Check sheet for the modelled part. Datum: model origin and axes. Units: mm. Face numbers are marked on the shaded views. A direction names the side the tool comes from. Give positions to 0.01 mm unless a question says otherwise; leave off trailing zeros. Order: outer loops, then holes, each group sorted by start corner. A loop starts at its lowest first (then second) coordinate and runs counter-clockwise, first axis right, second up. Notation, with made-up numbers: (9, -7) -> (46, -7) arc R15 cw to (46, -3) -> close; hole circle Ø4 at (15, 14.5). An arc over 180 degrees is marked (long way). One line per question, with ' | ' between items. Start each with the question number.
from build123d import *

# Parameters (mm, degrees)
BOSS_EXTRUDE1_DEPTH = 3
CUT_EXTRUDE1_REACH  = 5
SKETCH3_W           = 2.8
SKETCH3_H           = 2.8


with BuildPart() as part:
    # Sketch1 → Boss-Extrude1 (new body)
    with BuildSketch(Plane(origin=(0, 0, 0), x_dir=(1, 0, 0), z_dir=(0, 1, 0))):
        Polygon((0, 14.43375673), (-12.5, -7.216878365), (12.5, -7.216878365), align=None)
    extrude(amount=BOSS_EXTRUDE1_DEPTH)

    # Sketch3 → Cut-Extrude1 (cut, up to next)
    with BuildSketch(Plane(origin=(0, 3, 0), x_dir=(1, 0, 0), z_dir=(0, 1, 0)), mode=Mode.PRIVATE) as cut_extrude1_sk1:
        Polygon((6.95, 2.396003617), (4.525128869, 0.996003617), (3.125128869, 3.420874748), (5.55, 4.820874748), align=None)
    cut_extrude1_tool1 = extrude(cut_extrude1_sk1.sketch, amount=-CUT_EXTRUDE1_REACH, mode=Mode.PRIVATE) & part.part
    add(cut_extrude1_tool1.solids().sort_by_distance((5.037564, 3, -2.908439))[0], mode=Mode.SUBTRACT)
    # Sketch3 → Cut-Extrude1 (cut, up to next)
    with BuildSketch(Plane(origin=(0, 3, 0), x_dir=(1, 0, 0), z_dir=(0, 1, 0)), mode=Mode.PRIVATE) as cut_extrude1_sk2:
        Polygon((-6.95, 2.396003617), (-4.525128869, 0.996003617), (-3.125128869, 3.420874748), (-5.55, 4.820874748), align=None)
    cut_extrude1_tool2 = extrude(cut_extrude1_sk2.sketch, amount=-CUT_EXTRUDE1_REACH, mode=Mode.PRIVATE) & part.part
    add(cut_extrude1_tool2.solids().sort_by_distance((-5.037564, 3, -2.908439))[0], mode=Mode.SUBTRACT)
    # Sketch3 → Cut-Extrude1 (cut, up to next)
    with BuildSketch(Plane(origin=(0, 3, 0), x_dir=(1, 0, 0), z_dir=(0, 1, 0)), mode=Mode.PRIVATE) as cut_extrude1_sk3:
        with Locations((0, -5.816878365)):
            Rectangle(SKETCH3_W, SKETCH3_H)
    cut_extrude1_tool3 = extrude(cut_extrude1_sk3.sketch, amount=-CUT_EXTRUDE1_REACH, mode=Mode.PRIVATE) & part.part
    add(cut_extrude1_tool3.solids().sort_by_distance((0, 3, 5.816878))[0], mode=Mode.SUBTRACT)


solid = part.part
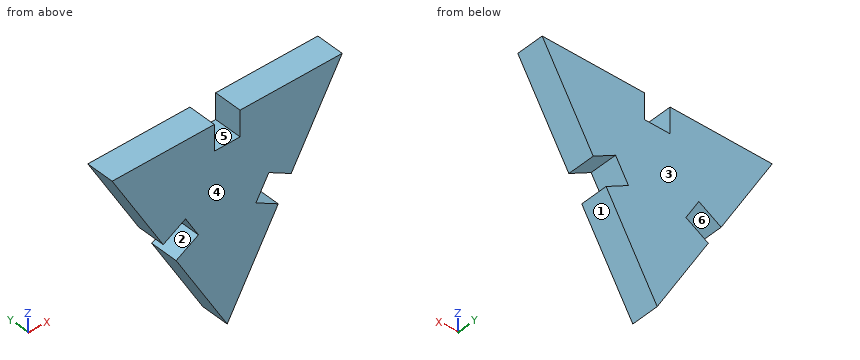
1. Cross-section at B-B on z = -2.75. Record the boundary of the cut face in (x, y), and give its area (3 significant figures).
2. Mould release check, pull along Z, two halves, no side actions. Record for the marked faces 1, 2 and 3: +Z half, -Z half, draft (parallel to the pull), parting line (faces both ways), or undercut.
3. Tool access check on the marked faces 4, 5 and 6. Record the directions out of +Z, -Z, +X, -X, +Y, -Y that give a thin tool (end or side, any length) a straight path to the whole face; none if there is none.
4. Go/stop test with flat-tipped pins: pin 1 (1.5 mm diameter, centred on y = 0.5, z = 0, fed in from +X); pin 2 (1.5 mm diameter, centred on x = 2, y = 2, fed in from -Z); pin 3 (0.8 mm diameter, centred on y = 2, z = 6, fed in from +X). Record where each tip stops, or that it passes through.
5. Scan lines: probe 1 along X at (y, z) = (2.65, -2); probe 2 along X at (y, z) = (2, -12); probe 3 along Z at (x, y) = (-3.75, 0.55). Record each from-to range of solid material in increasing order.
6. Cross-section at C-C on x = 10.5. Record the boundary of the cut face in (y, z), and give its area (3 significant figures).
7. Cross-section at A-A on y = 2. Record the boundary of the cut face in (x, z).
Response values:
1) outline: (-3.51, 0) -> (3.51, 0) -> (3.51, 3) -> (-3.51, 3) -> close | area: 21.1 mm²
2) face 1: -Z half | face 2: undercut | face 3: draft
3) face 4: +Z, -Z, +X, -X, -Y | face 5: +Z, +Y, -Y | face 6: +Y, -Y
4) pin 1: stops at x = 8.77 | pin 2: stops at z = -12.27 | pin 3: stops at x = 12.03
5) probe 1: x = -7.18 to -6.26, -3.95 to 3.95, 6.26 to 7.18 | probe 2: x = -1.41 to 1.41 | probe 3: z = -7.94 to -3.78, -2.34 to 7.22
6) outline: (0, 3.75) -> (3, 3.75) -> (3, 7.22) -> (0, 7.22) -> close | area: 10.4 mm²
7) outline: (-12.5, 7.22) -> (-6.95, -2.4) -> (-4.53, -1) -> (-3.13, -3.42) -> (-5.55, -4.82) -> (0, -14.43) -> (5.55, -4.82) -> (3.13, -3.42) -> (4.53, -1) -> (6.95, -2.4) -> (12.5, 7.22) -> (1.4, 7.22) -> (1.4, 4.42) -> (-1.4, 4.42) -> (-1.4, 7.22) -> close
